Can you work these out from the drawing? Everything is in mm from the part's minimum corner. A direction names the side the tool comes from. Round coordinates to 2 decimals unless told otherwise and drop trailing zeros. Write each loop counter-clockwise with the first axis right and the second up, starting at its lowest first coordinate (ties: lowest second). Pieces come first, ordered by that corner, then holes. Notation, with made-up numbers: (35, -1.75) -> (63, -1.75) arc R15 cw to (63, 19.25) -> close; hole circle Ø8 at (15, 19). An arc over 180 degrees is marked (long way). Put each result on its own line as item: value. Start each with the question number.
1. I need wall thicknesses on probe 1 along Y at (x, z) = (60, 66); probe 2 along X at (y, z) = (8.5, 55); probe 3 along Z at (x, y) = (24, 11.5). Which ranges of each line are inside material? Lowest first, please. Write a range as from..to.
2. Suppose I cut it at C-C (x = 25). Please give me the cut outline in (y, z).
3. We'd pull the mould along X, two halves only. Please class the marked faces 3, 4, 5 and 6: +X half, -X half, draft (parallel to the pull), parting line (faces both ways), or undercut.
4. Suppose I cut it at B-B (y = 10). Please give me the cut outline in (x, z), then the cut area to 3 significant figures.
5. Suppose I cut it at A-A (z = 55). Please give me the cut outline in (x, y).
6. For pin 1 (10 mm diameter, centred on y = 8, z = 20, fed in from +X), with a flat end and sliding along its axis, tell me the tip position at first contact or that it passes through.
7. Which directions (+Z, -Z, +X, -X, +Y, -Y) give clear straight access to the entire face, cutting with the end or side of a thin tool? Please do the marked faces 1 and 2.
8. Suppose I cut it at D-D (z = 20). Please give me the cut outline in (x, y).
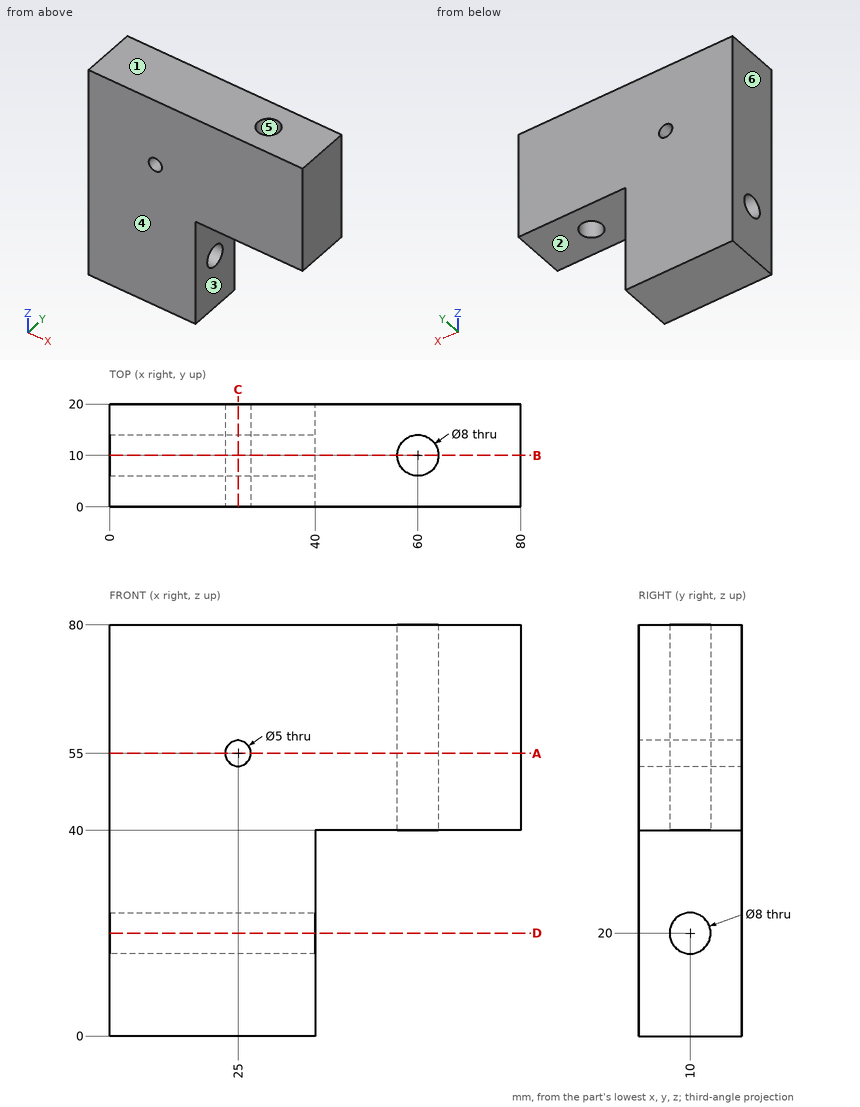
Verdict:
1. probe 1: y = 0..6, 14..20
1. probe 2: x = 0..22.5, 27.5..56.29, 63.71..80
1. probe 3: z = 0..16.29, 23.71..52.71, 57.29..80
2. outline: (0, 0) -> (20, 0) -> (20, 52.5) -> (0, 52.5) -> close; (0, 57.5) -> (20, 57.5) -> (20, 80) -> (0, 80) -> close; hole circle Ø8 at (10, 20)
3. face 3: +X half
3. face 4: draft
3. face 5: undercut
3. face 6: -X half
4. outline: (0, 0) -> (40, 0) -> (40, 16) -> (0, 16) -> close; (0, 24) -> (40, 24) -> (40, 40) -> (56, 40) -> (56, 80) -> (0, 80) -> close; (64, 40) -> (80, 40) -> (80, 80) -> (64, 80) -> close; hole circle Ø5 at (25, 55)
4. area: 4,140 mm^2
5. outline: (0, 0) -> (22.5, 0) -> (22.5, 20) -> (0, 20) -> close; (27.5, 0) -> (80, 0) -> (80, 20) -> (27.5, 20) -> close; hole circle Ø8 at (60, 10)
6. pin 1: stops at x = 40
7. face 1: +Z, +X, -X, +Y, -Y
7. face 2: -Z, +X, +Y, -Y
8. outline: (0, 0) -> (40, 0) -> (40, 6) -> (0, 6) -> close; (0, 14) -> (40, 14) -> (40, 20) -> (0, 20) -> close
